Can you work these out from the model? Positions are in its coordinate system, mm. Face numbers are marked on the shaded views. Round coordinates to 2 decimals unless told otherwise and drop trailing zeros. Write each loop counter-clockwise with the first axis right and the second up, starting at its lowest first coordinate (ties: lowest second). Pieces come first, ordered by that corner, then holes.
Q1. We'd pull the mould along Z, two halves only. Please class the marked faces 1 and 2: +Z half, -Z half, draft (parallel to the pull), parting line (faces both ways), or undercut.
Q2. I'm going to push flat-ended pins straight in: pin 1 Ø2.5 at (x, z) = (1.5, -2.5) entering from -Y; pin 2 Ø5.5 at (y, z) = (25, -61.5) entering from -X; pin 3 Ø5.5 at (y, z) = (1.5, -12.5) entering from +X; pin 4 Ø12 at (x, z) = (-2, -49) entering from -Y. Where does each tip first touch, or does it pass through?
Q3. If we section it at C-C (y = 19): Please give me the cut outline in (x, z).
Q4. If we section it at A-A (z = -29): Please give me the cut outline in (x, y), plus the area to 3 significant figures.
Q5. If we section it at B-B (x = -20): Please give me the cut outline in (y, z), plus the area to 3 significant figures.
Q6. Please list where these lines run through material, in increasing order: line 1 along X through (y, z) = (41, -49); line 2 along Y through (x, z) = (-5, 43.5); line 3 along Z through (x, y) = (-3, 18.5).
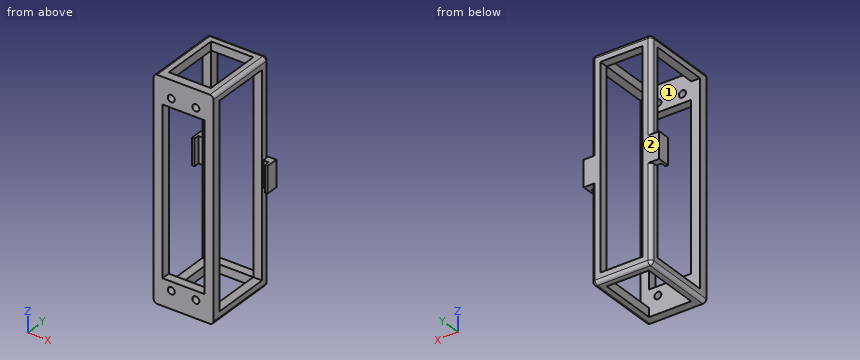
Autodesk Inventor part; units mm, degrees
ref_plane "YZ Plane" through (0, 0, 0) normal (1, 0, 0) x (0, 1, 0)
ref_plane "XZ Plane" through (0, 0, 0) normal (0, 1, 0) x (-1, 0, 0)
ref_plane "XY Plane" through (0, 0, 0) normal (0, 0, 1) x (1, 0, 0)
sketch "Sketch2" plane through (0, 0, 0) normal (0, 1, 0) x (-1, 0, 0)
  line L0 (34.7144, 60.4703) -> (0.7144, 60.4703)
  line L1 (0.7144, 60.4703) -> (0.7144, -63.8297)
  line L2 (0.7144, -63.8297) -> (34.7144, -63.8297)
  line L3 (34.7144, -63.8297) -> (34.7144, 60.4703)
  point P0 (0, 0)
  dimension "d0" = 124.3
  dimension "d1" = 34
extrude "Extrusion1" add sketch "Sketch2" along normal blind 43.5
sketch "Sketch3" plane through (0, 43.5, 0) normal (0, 1, 0) x (1, 0, 0)
  line L0 (-34.7144, -60.4703) -> (-0.7144, -60.4703) construction
  line L1 (-0.7144, -60.4703) -> (-0.7144, 63.8297) construction
  line L2 (-0.7144, 63.8297) -> (-34.7144, 63.8297) construction
  line L3 (-34.7144, 63.8297) -> (-34.7144, -60.4703) construction
  line L4 (-29.7144, 58.8297) -> (-5.7144, 58.8297)
  line L5 (-5.7144, 58.8297) -> (-5.7144, -55.4703)
  line L6 (-5.7144, -55.4703) -> (-29.7144, -55.4703)
  line L7 (-29.7144, -55.4703) -> (-29.7144, 58.8297)
  point P0 (0, 0)
  dimension "d4" = 114.3
  dimension "d5" = 24
  dimension "d6" = 5
  dimension "d7" = 5
  dimension "d8" = 5
  dimension "d9" = 5
extrude "Extrusion2" cut sketch "Sketch3" against normal blind 38.5
sketch "Sketch4" plane through (-0.7144, 0, 60.4703) normal (1, 0, 0) x (0, 0, -1)
  line L0 (124.3, 0) -> (124.3, 43.5) construction
  line L1 (0, 43.5) -> (124.3, 43.5) construction
  line L2 (54.65, 43.5) -> (69.65, 43.5)
  line L3 (69.65, 43.5) -> (69.65, 36.5)
  line L4 (69.65, 36.5) -> (54.65, 36.5)
  line L5 (54.65, 36.5) -> (54.65, 43.5)
  point P0 (60.4703, 0)
  dimension "d12" = 15
  dimension "d13" = 7
  dimension "d14" = 0
  dimension "d15" = 54.65
extrude "Extrusion3" add sketch "Sketch4" along normal blind 4.5
sketch "Sketch5" plane through (-34.7144, 0, -63.8297) normal (-1, 0, 0) x (0, 0, 1)
  line L0 (124.3, 0) -> (124.3, 43.5) construction
  line L1 (0, 43.5) -> (124.3, 43.5) construction
  line L2 (54.65, 43.5) -> (69.65, 43.5)
  line L3 (69.65, 43.5) -> (69.65, 36.5)
  line L4 (69.65, 36.5) -> (54.65, 36.5)
  line L5 (54.65, 36.5) -> (54.65, 43.5)
  point P0 (63.8297, 0)
  dimension "d18" = 7
  dimension "d19" = 15
  dimension "d20" = 0
  dimension "d21" = 54.65
extrude "Extrusion4" add sketch "Sketch5" along normal blind 4.5
sketch "Sketch6" plane through (-34.7144, 36.5, -9.1797) normal (0, -1, 0) x (1, 0, 0)
  line L0 (0, 15) -> (0, 0) construction
  line L1 (0, 15) -> (-4.5, 15) construction
  line L2 (-3, 0) -> (0, 0)
  line L3 (0, 0) -> (0, 15)
  line L4 (0, 15) -> (-3, 15)
  line L5 (-3, 15) -> (-3, 0)
  point P0 (34.7144, 9.1797)
  dimension "d24" = 15
  dimension "d25" = 3
  dimension "d26" = 0
  dimension "d27" = 0
extrude "Extrusion5" cut sketch "Sketch6" against normal blind 3
sketch "Sketch7" plane through (-0.7144, 36.5, -9.1797) normal (0, -1, 0) x (1, 0, 0)
  line L0 (0, 0) -> (0, 15) construction
  line L1 (0, 15) -> (4.5, 15) construction
  line L2 (0, 15) -> (3, 15)
  line L3 (3, 15) -> (3, 0)
  line L4 (3, 0) -> (0, 0)
  line L5 (0, 0) -> (0, 15)
  point P0 (0.7144, 9.1797)
  dimension "d30" = 15
  dimension "d31" = 3
  dimension "d32" = 0
  dimension "d33" = 0
extrude "Extrusion6" cut sketch "Sketch7" against normal blind 3
sketch "Sketch8" plane through (-34.7144, 0, 60.4703) normal (0, 0, 1) x (1, 0, 0)
  line L0 (0, 0) -> (34, 0) construction
  line L1 (34, 0) -> (34, 43.5) construction
  line L2 (0, 43.5) -> (34, 43.5) construction
  line L3 (0, 0) -> (0, 43.5) construction
  line L4 (5, 38.5) -> (29, 38.5)
  line L5 (29, 38.5) -> (29, 5)
  line L6 (29, 5) -> (5, 5)
  line L7 (5, 5) -> (5, 38.5)
  point P0 (34.7144, 0)
  dimension "d36" = 33.5
  dimension "d37" = 24
  dimension "d38" = 5
  dimension "d39" = 5
  dimension "d40" = 5
  dimension "d41" = 5
extrude "Extrusion7" cut sketch "Sketch8" against normal blind 124.3
sketch "Sketch9" plane through (-0.7144, 0, 60.4703) normal (1, 0, 0) x (0, 0, -1)
  line L0 (0, 0) -> (0, 43.5) construction
  line L1 (0, 0) -> (124.3, 0) construction
  line L2 (124.3, 0) -> (124.3, 43.5) construction
  line L3 (69.65, 43.5) -> (124.3, 43.5) construction
  line L4 (5, 38.5) -> (119.3, 38.5)
  line L5 (119.3, 38.5) -> (119.3, 5)
  line L6 (119.3, 5) -> (5, 5)
  line L7 (5, 5) -> (5, 38.5)
  point P0 (60.4703, 0)
  dimension "d44" = 114.3
  dimension "d45" = 33.5
  dimension "d46" = 5
  dimension "d47" = 5
  dimension "d48" = 5
  dimension "d49" = 5
extrude "Extrusion8" cut sketch "Sketch9" against normal blind 34
sketch "Sketch11" plane through (0, 0, 0) normal (0, -1, 0) x (1, 0, 0)
  line L0 (-34.7144, 60.4703) -> (-0.7144, 60.4703) construction
  line L1 (-34.7144, -63.8297) -> (-34.7144, 60.4703) construction
  line L2 (-0.7144, -63.8297) -> (-34.7144, -63.8297) construction
  line L3 (-0.7144, 60.4703) -> (-0.7144, -63.8297) construction
  circle A0 centre (-24.7144, -53.8297) radius 2
  circle A1 centre (-10.7144, -53.8297) radius 2
  circle A2 centre (-24.7144, 50.4703) radius 2
  circle A3 centre (-10.7144, 50.4703) radius 2
  line L4 (-29.7144, -48.8297) -> (-5.7144, -48.8297)
  line L5 (-5.7144, -48.8297) -> (-5.7144, 45.4703)
  line L6 (-5.7144, 45.4703) -> (-29.7144, 45.4703)
  line L7 (-29.7144, 45.4703) -> (-29.7144, -48.8297)
  point P0 (0, 0)
  dimension "d52" = 4
  dimension "d53" = 10
  dimension "d54" = 10
  dimension "d55" = 4
  dimension "d56" = 10
  dimension "d57" = 10
  dimension "d58" = 4
  dimension "d59" = 10
  dimension "d60" = 10
  dimension "d61" = 4
  dimension "d62" = 10
  dimension "d63" = 10
  dimension "d66" = 94.3
  dimension "d67" = 24
  dimension "d68" = 5
  dimension "d69" = 5
  dimension "d70" = 5
  dimension "d71" = 5
extrude "Extrusion9" cut sketch "Sketch11" against normal blind 5 contours A0 | A1 | A2 | A3
sketch "Sketch12" plane through (0, 0, 0) normal (0, -1, 0) x (1, 0, 0)
  circle A0 centre (-24.7144, 50.4703) radius 2 construction
  circle A1 centre (-24.7144, -53.8297) radius 2 construction
  line L0 (-34.7144, -63.8297) -> (-34.7144, 60.4703) construction
  line L1 (-0.7144, 60.4703) -> (-0.7144, -63.8297) construction
  line L2 (-29.7144, -48.8297) -> (-5.7144, -48.8297)
  line L3 (-5.7144, -48.8297) -> (-5.7144, 45.4703)
  line L4 (-5.7144, 45.4703) -> (-29.7144, 45.4703)
  line L5 (-29.7144, 45.4703) -> (-29.7144, -48.8297)
  point P0 (0, 0)
  dimension "d72" = 94.3
  dimension "d73" = 24
  dimension "d74" = 5
  dimension "d75" = 5
  dimension "d76" = 5
  dimension "d77" = 5
extrude "Extrusion10" cut sketch "Sketch12" against normal blind 5
fillet "Fillet1" radius 2 10 edges at (-34.7144, 43.5, -36.5047) (-34.7144, 43.5, 33.1453) (-17.7144, 43.5, 60.4703) (-0.7144, 43.5, 33.1453) (-0.7144, 43.5, -36.5047) (-17.7144, 43.5, -63.8297) (-34.7144, 21.75, 60.4703) (-0.7144, 21.75, 60.4703) (-0.7144, 21.75, -63.8297) (-34.7144, 21.75, -63.8297)
properties part number "Battery Case"
A:
1. face 1: undercut
1. face 2: draft
2. pin 1: stops at y = 36.5
2. pin 2: stops at x = -34.71
2. pin 3: stops at x = -0.71
2. pin 4: stops at y = 0
3. outline: (-34.71, -61.83) arc R2 ccw to (-32.71, -63.83) - (-29.71, -63.83) - (-29.71, -58.83) - (-34.71, -58.83) - close; (-34.71, 55.47) - (-29.71, 55.47) - (-29.71, 60.47) - (-32.71, 60.47) arc R2 ccw to (-34.71, 58.47) - close; (-5.71, -63.83) - (-2.71, -63.83) arc R2 ccw to (-0.71, -61.83) - (-0.71, -58.83) - (-5.71, -58.83) - close; (-5.71, 55.47) - (-0.71, 55.47) - (-0.71, 58.47) arc R2 ccw to (-2.71, 60.47) - (-5.71, 60.47) - close
4. outline: (-34.71, 0) - (-29.71, 0) - (-29.71, 5) - (-34.71, 5) - close; (-34.71, 38.5) - (-29.71, 38.5) - (-29.71, 43.5) - (-32.71, 43.5) arc R2 ccw to (-34.71, 41.5) - close; (-5.71, 0) - (-0.71, 0) - (-0.71, 5) - (-5.71, 5) - close; (-5.71, 38.5) - (-0.71, 38.5) - (-0.71, 41.5) arc R2 ccw to (-2.71, 43.5) - (-5.71, 43.5) - close
4. area: 98.3 mm2
5. outline: (0, -63.83) - (5, -63.83) - (5, -48.83) - (0, -48.83) - close; (0, 45.47) - (5, 45.47) - (5, 60.47) - (0, 60.47) - close; (38.5, -63.83) - (41.5, -63.83) arc R2 ccw to (43.5, -61.83) - (43.5, -58.83) - (38.5, -58.83) - close; (38.5, 55.47) - (43.5, 55.47) - (43.5, 58.47) arc R2 ccw to (41.5, 60.47) - (38.5, 60.47) - close
5. area: 198 mm2
6. line 1: x = -34.71 to -29.71, -5.71 to -0.71
6. line 2: y = 0 to 5, 38.5 to 43.5
6. line 3: z = -63.83 to -58.83, 55.47 to 60.47
